Design review of the part built by this model. Coordinates are the model's own, in mm. Coordinates: 2 decimals unless noted, no trailing zeros. Write each loop counter-clockwise with the first axis right and the second up, starting at its lowest first coordinate (ties: lowest second). Pieces come first, ordered by that corner, then holes.
```python
from build123d import *

# Parameters (mm, degrees)
ESBO_O1_W                = 50
ESBO_O1_H                = 50
ESBO_O1_R                = 11
ESBO_O1_R_2              = 1.5
RESSALTO_EXTRUS_O1_DEPTH = 10
ESBO_O2_W                = 50
ESBO_O2_H                = 2.5
RESSALTO_EXTRUS_O2_DEPTH = 50
ESBO_O3_R                = 1.5
CORTE_EXTRUS_O1_DEPTH    = 101
ESBO_O1_2_W              = 50
ESBO_O1_2_H              = 50
ESBO_O1_2_R              = 11
ESBO_O1_2_R_2            = 1.5
RESSALTO_EXTRUS_O3_DEPTH = 4
ESBO_O5_W                = 50
ESBO_O5_H                = 5
CORTE_EXTRUS_O2_DEPTH    = 47.5
FILETE2_R                = 2


with BuildPart() as part:
    # Esboço1 → Ressalto-extrusão1 (new body)
    with BuildSketch(Plane.XY):
        with Locations((25, -25)):
            Rectangle(ESBO_O1_W, ESBO_O1_H)
        with Locations((25, -25)):
            Circle(ESBO_O1_R, mode=Mode.SUBTRACT)
        with Locations((8.5, -8.5)):
            Circle(ESBO_O1_R_2, mode=Mode.SUBTRACT)
        with Locations((41.546450715, -8.453549285)):
            Circle(ESBO_O1_R_2, mode=Mode.SUBTRACT)
        with Locations((41.546450715, -41.546450715)):
            Circle(ESBO_O1_R_2, mode=Mode.SUBTRACT)
        with Locations((8.5, -41.5)):
            Circle(ESBO_O1_R_2, mode=Mode.SUBTRACT)
    extrude(amount=RESSALTO_EXTRUS_O1_DEPTH)

    # Esboço2 → Ressalto-extrusão2 (add)
    with BuildSketch(Plane.XY):
        with Locations((25, -48.75)):
            Rectangle(ESBO_O2_W, ESBO_O2_H)
    extrude(amount=RESSALTO_EXTRUS_O2_DEPTH)

    # Esboço3 → Corte-extrusão1 (cut)
    with BuildSketch(Plane(origin=(0, 0, 0), x_dir=(1, 0, 0), z_dir=(0, 1, 0))):
        with Locations((4, -37)):
            Circle(ESBO_O3_R)
        with Locations((4, -44)):
            Circle(ESBO_O3_R)
        with Locations((11, -44)):
            Circle(ESBO_O3_R)
        with Locations((18, -44)):
            Circle(ESBO_O3_R)
        with Locations((25, -44)):
            Circle(ESBO_O3_R)
        with Locations((32, -44)):
            Circle(ESBO_O3_R)
        with Locations((39, -44)):
            Circle(ESBO_O3_R)
        with Locations((46, -44)):
            Circle(ESBO_O3_R)
        with Locations((46, -37)):
            Circle(ESBO_O3_R)
        with Locations((39, -37)):
            Circle(ESBO_O3_R)
        with Locations((32, -37)):
            Circle(ESBO_O3_R)
        with Locations((25, -37)):
            Circle(ESBO_O3_R)
        with Locations((18, -37)):
            Circle(ESBO_O3_R)
        with Locations((11, -37)):
            Circle(ESBO_O3_R)
        with Locations((4, -30)):
            Circle(ESBO_O3_R)
        with Locations((11, -30)):
            Circle(ESBO_O3_R)
        with Locations((18, -30)):
            Circle(ESBO_O3_R)
        with Locations((32, -30)):
            Circle(ESBO_O3_R)
        with Locations((25, -30)):
            Circle(ESBO_O3_R)
        with Locations((39, -30)):
            Circle(ESBO_O3_R)
        with Locations((46, -30)):
            Circle(ESBO_O3_R)
        with Locations((46, -23)):
            Circle(ESBO_O3_R)
        with Locations((39, -23)):
            Circle(ESBO_O3_R)
        with Locations((32, -23)):
            Circle(ESBO_O3_R)
        with Locations((18, -23)):
            Circle(ESBO_O3_R)
        with Locations((25, -23)):
            Circle(ESBO_O3_R)
        with Locations((11, -23)):
            Circle(ESBO_O3_R)
        with Locations((4, -23)):
            Circle(ESBO_O3_R)
        with Locations((4, -16)):
            Circle(ESBO_O3_R)
        with Locations((11, -16)):
            Circle(ESBO_O3_R)
        with Locations((18, -16)):
            Circle(ESBO_O3_R)
        with Locations((25, -16)):
            Circle(ESBO_O3_R)
        with Locations((32, -16)):
            Circle(ESBO_O3_R)
        with Locations((39, -16)):
            Circle(ESBO_O3_R)
        with Locations((46, -16)):
            Circle(ESBO_O3_R)
    extrude(amount=-CORTE_EXTRUS_O1_DEPTH, mode=Mode.SUBTRACT)

    # Esboço1<2> → Ressalto-extrusão3 (add)
    with BuildSketch(Plane.XY):
        with Locations((25, -25)):
            Rectangle(ESBO_O1_2_W, ESBO_O1_2_H)
        with Locations((25, -25)):
            Circle(ESBO_O1_2_R, mode=Mode.SUBTRACT)
        with Locations((8.5, -8.5)):
            Circle(ESBO_O1_2_R_2, mode=Mode.SUBTRACT)
        with Locations((41.546450715, -8.453549285)):
            Circle(ESBO_O1_2_R_2, mode=Mode.SUBTRACT)
        with Locations((41.546450715, -41.546450715)):
            Circle(ESBO_O1_2_R_2, mode=Mode.SUBTRACT)
        with Locations((8.5, -41.5)):
            Circle(ESBO_O1_2_R_2, mode=Mode.SUBTRACT)
    extrude(amount=RESSALTO_EXTRUS_O3_DEPTH)

    # Esboço5 → Corte-extrusão2 (cut)
    with BuildSketch(Plane(origin=(0, 0, 0), x_dir=(1, 0, 0), z_dir=(0, 1, 0))):
        with Locations((25, -7.5)):
            Rectangle(ESBO_O5_W, ESBO_O5_H)
    extrude(amount=-CORTE_EXTRUS_O2_DEPTH, mode=Mode.SUBTRACT)

    # Filete2
    filete2_edges = [part.edges().sort_by_distance(p)[0] for p in [
        (25, -47.5, 5),
    ]]
    fillet(filete2_edges, radius=FILETE2_R)


solid = part.part
```
(1) Wall thickness on line 1 (Z direction, x = 32, y = -49); line 2 (Y direction, x = 8.5, z = 2.4); line 3 (Y direction, x = 4.5, z = 31.5): over which ranges is each line inside the solid? List them lowest first.
(2) Consider section A-A (z = 16). State how many separate pieces and enclosed holes the cut face has, plus the area to 3 significant figures.
(3) Consider section C-C (x = 8.5). Give the boundary of the cut face in (y, z).
(4) Consider section B-B (x = 39). Give the boundary of the cut face in (y, z).
(5) Insertion check: pin 1 Ø4 at (x, z) = (18, 44) entering from +Y; pin 2 Ø8 at (x, y) = (44, -28.5) entering from +Z. Each pin has a flat end and moves straight along its axis. Give the tip position at first contact, or say it passes through.
(6) Mouldability with a two-part tool opening along Y and no side actions: class faces 1 (the cylindrical face through (10.675, -48.732, 45.464)), 2 (the cylindrical face through (40.36, -9.37, 2.46)) as +Y half, -Y half, draft (parallel to the pull), parting line (faces both ways), or undercut.
(7) Consider section D-D (y = -32.5). Give the boundary of the cut face in (x, z).
Results:
1. line 1: z = 0 to 14.5, 17.5 to 21.5, 24.5 to 28.5, 31.5 to 35.5, 38.5 to 42.5, 45.5 to 50
1. line 2: y = -50 to -43, -40 to -10, -7 to 0
1. line 3: y = -50 to -47.5
2. separate pieces: 8
2. enclosed holes: 0
2. area: 72.5 mm2
3. outline: (-50, 0) - (-43, 0) - (-43, 5) - (-45.5, 5) arc R2 cw to (-47.5, 7) - (-47.5, 50) - (-50, 50) - close; (-40, 0) - (-10, 0) - (-10, 5) - (-40, 5) - close; (-7, 0) - (0, 0) - (0, 5) - (-7, 5) - close
4. outline: (-50, 0) - (0, 0) - (0, 5) - (-45.5, 5) arc R2 cw to (-47.5, 7) - (-47.5, 14.5) - (-50, 14.5) - close; (-50, 17.5) - (-47.5, 17.5) - (-47.5, 21.5) - (-50, 21.5) - close; (-50, 24.5) - (-47.5, 24.5) - (-47.5, 28.5) - (-50, 28.5) - close; (-50, 31.5) - (-47.5, 31.5) - (-47.5, 35.5) - (-50, 35.5) - close; (-50, 38.5) - (-47.5, 38.5) - (-47.5, 42.5) - (-50, 42.5) - close; (-50, 45.5) - (-47.5, 45.5) - (-47.5, 50) - (-50, 50) - close
5. pin 1: stops at y = -47.5
5. pin 2: stops at z = 5
6. face 1: draft
6. face 2: undercut
7. outline: (0, 0) - (16.95, 0) - (16.95, 5) - (0, 5) - close; (33.05, 0) - (50, 0) - (50, 5) - (33.05, 5) - close
